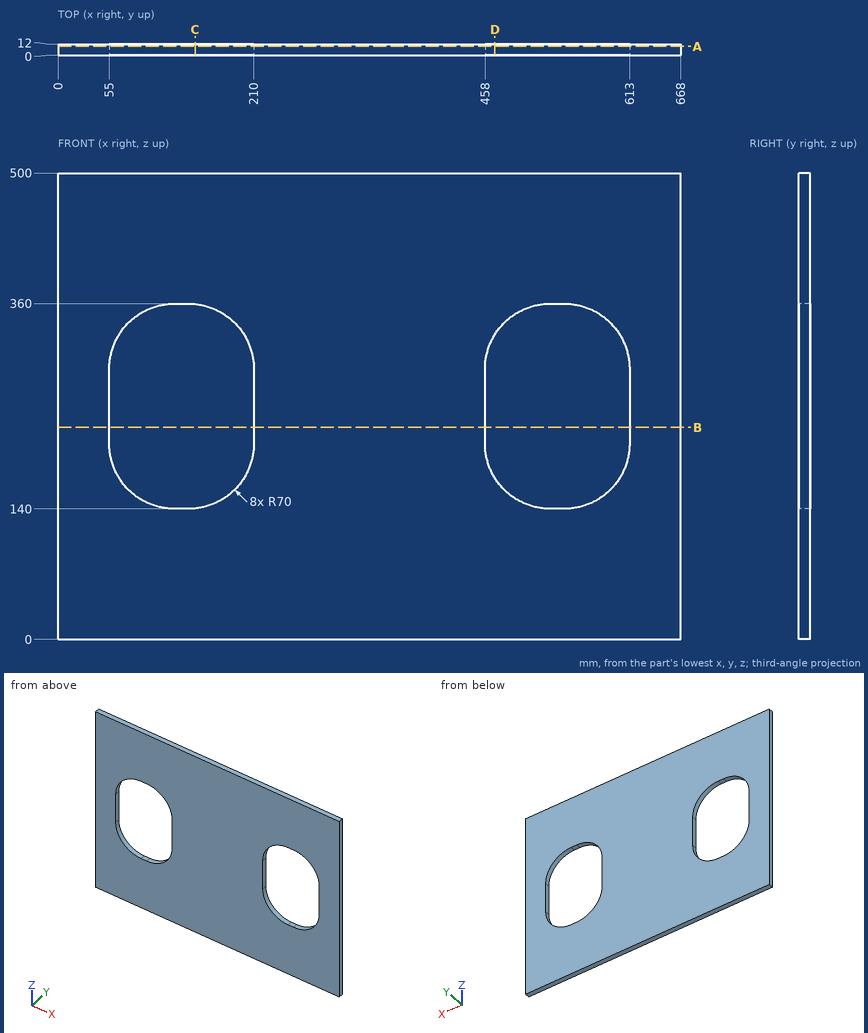
Verification items for this drawing (mm, ordinates from the low corner). Give positions to 0.01 mm unless a question says otherwise; leave off trailing zeros. Write each loop counter-clockwise with the first axis right and the second up, starting at its lowest first coordinate (ties: lowest second). Pieces come first, ordered by that corner, then holes. Notation, with made-up numbers: (83, 56.25) -> (141, 56.25) arc R27 ccw to (141, 82.25) -> close; hole circle Ø4 at (11.25, -16). An arc over 180 degrees is marked (long way). Use CSV: the item, a comma, the result in double quotes. Start each with the question number.
Q1. Cross-section at B-B on z = 227.5. Enter the section's corners in (x, y).
Q2. Scan lines: line 1 along X through (y, z) = (11, 275); line 2 along X through (y, z) = (11.25, 338); line 3 along Z through (x, y) = (479.5, 9). Record each from-to range of solid material in increasing order.
Q3. Cross-section at C-C on x = 147. Enter the section's corners in (y, z).
Q4. Cross-section at A-A on y = 9.5. Enter the section's corners in (x, z), and give its area (3 significant figures).
Q5. Cross-section at D-D on x = 468.5. Enter the section's corners in (y, z).
Q6. Depth check by flat-ended pin: P1, Ø1.5, axis at x = 117, z = 406.5, coming from the -Y side. Enter the tip coordinate at first touch or a pass-through.
Working result:
1,outline,"(0, 0) -> (55, 0) -> (55, 12) -> (0, 12) -> close; (210, 0) -> (458, 0) -> (458, 12) -> (210, 12) -> close; (613, 0) -> (668, 0) -> (668, 12) -> (613, 12) -> close"
2,line 1,"x = 0 to 55, 210 to 458, 613 to 668"
2,line 2,"x = 0 to 74.05, 190.95 to 477.05, 593.95 to 668"
2,line 3,"z = 0 to 159.52, 340.48 to 500"
3,outline,"(0, 0) -> (12, 0) -> (12, 140.35) -> (0, 140.35) -> close; (0, 359.65) -> (12, 359.65) -> (12, 500) -> (0, 500) -> close"
4,outline,"(0, 0) -> (668, 0) -> (668, 500) -> (0, 500) -> close; hole (55, 210) arc R70 ccw to (125, 140) -> (140, 140) arc R70 ccw to (210, 210) -> (210, 290) arc R70 ccw to (140, 360) -> (125, 360) arc R70 ccw to (55, 290) -> close; hole (458, 210) arc R70 ccw to (528, 140) -> (543, 140) arc R70 ccw to (613, 210) -> (613, 290) arc R70 ccw to (543, 360) -> (528, 360) arc R70 ccw to (458, 290) -> close"
4,area,"274,000 mm^2"
5,outline,"(0, 0) -> (12, 0) -> (12, 173.13) -> (0, 173.13) -> close; (0, 326.87) -> (12, 326.87) -> (12, 500) -> (0, 500) -> close"
6,P1,"stops at y = 0"
